from build123d import *
from build123d import SkipClean  # not in build123d's __all__

# Parameters (mm, degrees)
F0_R      = 3.1
F0_R_2    = 1
F1_DEPTH  = 3
F2_DEPTH  = 6
F3_W      = 4
F3_H      = 10
F4_DEPTH  = 15
F5_R      = 1.75
F6_DEPTH  = 25
F8_DEPTH  = 2.5
F9_R      = 4.99999
F10_W     = 6
F10_H     = 0.4
F11_DEPTH = 25


# Not quite as in the source:
# - a fillet or chamfer is up to 0.001 mm smaller than in the source, because OpenCascade refuses the exact size
# - after a boolean that leaves OpenCascade's solid faulty, fix() repairs it


with BuildPart() as f1:
    # F0 (on Top) → F1 (new body)
    with BuildSketch(Plane.XY):
        with BuildLine():
            ThreePointArc((0, -5), (3.5355339059, -3.5355339059), (5, 0))
            ThreePointArc((5, 0), (3.5355339059, 3.5355339059), (0, 5))
            ThreePointArc((0, 5), (-5, 0), (0, -5))
        make_face()
        Circle(F0_R, mode=Mode.SUBTRACT)
        Circle(F0_R)
        Circle(F0_R_2, mode=Mode.SUBTRACT)
        with BuildLine():
            ThreePointArc((0, -5), (-5, 0), (0, 5))
            Line((0, 5), (-13.260579668, 5))
            Line((-13.260579668, 5), (-13.260579668, -5))
            Line((-13.260579668, -5), (0, -5))
        make_face()
        Circle(F0_R_2)
    extrude(amount=-F1_DEPTH)

    # F0 (on Top) → F2 (join)
    with BuildSketch(Plane.XY):
        with BuildLine():
            ThreePointArc((0, -5), (3.5355339059, -3.5355339059), (5, 0))
            ThreePointArc((5, 0), (3.5355339059, 3.5355339059), (0, 5))
            ThreePointArc((0, 5), (-5, 0), (0, -5))
        make_face()
        Circle(F0_R, mode=Mode.SUBTRACT)
    with SkipClean():  # cleaning this boolean's faces spoils the solid; the shape is the same uncleaned
        extrude(amount=F2_DEPTH)

    # F3 (on face) → F4 (join)
    with BuildSketch(Plane.XY):
        with Locations((-11.260579668, 0)):
            Rectangle(F3_W, F3_H)
    extrude(amount=F4_DEPTH)

    add(f1.part.fix(), mode=Mode.REPLACE)

    # F5 (on face) → F6 (cut)
    with BuildSketch(Plane.YZ.offset(-9.260579668)):
        with Locations((0, 10.6251845136)):
            Circle(F5_R)
    extrude(amount=-F6_DEPTH, mode=Mode.SUBTRACT)

    # F7 (on face) → F8 (cut)
    with BuildSketch(Plane.YZ.offset(-9.260579668)):
        Polygon((0, 7.3342879792), (2.85, 8.9797362464), (2.85, 12.2706327808), (0, 13.916081048), (-2.85, 12.2706327808), (-2.85, 8.9797362464), align=None)
    extrude(amount=-F8_DEPTH, mode=Mode.SUBTRACT)

    # F9 (radius 5 in the source; OpenCascade refuses exactly that, so slightly less here)
    f9_edges = [f1.edges().sort_by_distance(p)[0] for p in [
        (-11.26058, -5, 15),
        (-11.26058, 5, 15),
    ]]
    fillet(f9_edges, radius=F9_R)

    # F10 (on face) → F11 (cut)
    with BuildSketch(Plane.XY):
        Rectangle(F10_W, F10_H)
    extrude(amount=-F11_DEPTH, mode=Mode.SUBTRACT)


solid = f1.part
The listing builds one solid part. Answer for the finished solid, in the listing's coordinates (mm). A direction names the side the tool comes from. Coordinates: 2 decimals unless noted, no trailing zeros. Order: outer loops, then holes, each group sorted by start corner. A loop starts at its lowest first (then second) coordinate and runs counter-clockwise, first axis right, second up. Notation, with made-up numbers: (-1, 86.5) -> (8, 86.5) arc R16 ccw to (8, 100.5) -> close; hole circle Ø5 at (-21.5, -27.75). An arc over 180 degrees is marked (long way). Answer in a Markdown table with one row per item. Add a question column.
Item 1: Determine the mould class of faces 1 (the face through (-0.1, -3.3, 6)), 2 (the face through (-11, 3, 14)), 3 (the face through (-10.49, 1.41, 8.15)) for opening direction Y: +Y half, -Y half, draft (parallel to the pull), parting line (faces both ways), or undercut.
Item 2: Which of the six approach directions +Z, -Z, +X, -X, +Y, -Y give full straight-line access (tool end or side, diameter ignored) to faces 4 (the face through (-10, 5, 2)), 5 (the face through (-10, 2.85, 11)), 6 (the face through (1.43, -2.75, 2.96)), 7 (the face through (-9.261, 0, 6))?
Item 3: Each of these flat-tipped pins is pushed along its axis until it touches: P1, Ø6, axis at y = -1.5, z = 11, coming from the +X side; P2, Ø3.5, axis at x = 0.5, z = -1.5, coming from the +Y side; P3, Ø5, axis at x = 1, y = -0.5, coming from the +Z side; P4, Ø3, axis at y = 0, z = 10.63, coming from the -X side. Where does it stop, or does it pass through?
Item 4: Find section D-D (x = 0.5). Write down the section's boundary in (y, z), then the cut area to 3 significant figures.
Item 5: Find the intervals of material crossed by L1, parallel to X at y = -1.75, z = 4.75; L2, parallel to Y at x = 0, z = 2.6; L3, parallel to Z at x = -12.9, y = 0, in increasing order. Write a range as from..to.
Item 6: Find section C-C (y = 1.5). Write down the section's boundary in (x, z), then the cut area to 3 significant figures.
Item 7: Find section A-A (x = -4). Write down the section's boundary in (y, z), then the cut area to 3 significant figures.
Result set:
| question | item | result |
|---|---|---|
| 1 | face 1 | draft |
| 1 | face 2 | +Y half |
| 1 | face 3 | undercut |
| 2 | face 4 | +Z, -Z, +X, -X, +Y |
| 2 | face 5 | +X |
| 2 | face 6 | +Z |
| 2 | face 7 | +Z, +Y, -Y |
| 3 | P1 | stops at x = -9.26 |
| 3 | P2 | stops at y = 5 |
| 3 | P3 | stops at z = 6 |
| 3 | P4 | passes through |
| 4 | outline | (-4.97, -3) -> (-0.2, -3) -> (-0.2, 0) -> (-3.06, 0) -> (-3.06, 6) -> (-4.97, 6) -> close; (0.2, -3) -> (4.97, -3) -> (4.97, 6) -> (3.06, 6) -> (3.06, 0) -> (0.2, 0) -> close |
| 4 | area | 51.6 mm² |
| 5 | L1 | x = -13.26..-9.26, -4.68..-2.56, 2.56..4.68 |
| 5 | L2 | y = -5..-3.1, 3.1..5 |
| 5 | L3 | z = -3..8.88, 12.38..15 |
| 6 | outline | (-13.26, -3) -> (4.77, -3) -> (4.77, 6) -> (2.71, 6) -> (2.71, 0) -> (-2.71, 0) -> (-2.71, 6) -> (-4.77, 6) -> (-4.77, 0) -> (-9.26, 0) -> (-9.26, 8.2) -> (-11.76, 8.2) -> (-11.76, 9.72) -> (-13.26, 9.72) -> close; (-13.26, 11.53) -> (-11.76, 11.53) -> (-11.76, 13.05) -> (-9.26, 13.05) -> (-9.26, 14.77) -> (-13.26, 14.77) -> close |
| 6 | area | 123 mm² |
| 7 | outline | (-5, -3) -> (5, -3) -> (5, 0) -> (3, 0) -> (3, 6) -> (-3, 6) -> (-3, 0) -> (-5, 0) -> close |
| 7 | area | 66.0 mm² |
